Can you work these out from the drawing? Everything is in mm from the part's minimum corner. Coordinates: 2 decimals unless noted, no trailing zeros. Loops run counter-clockwise (first coordinate to the right, second up) from the corner with the lowest first, then second, coordinate; pieces in that order, holes last.
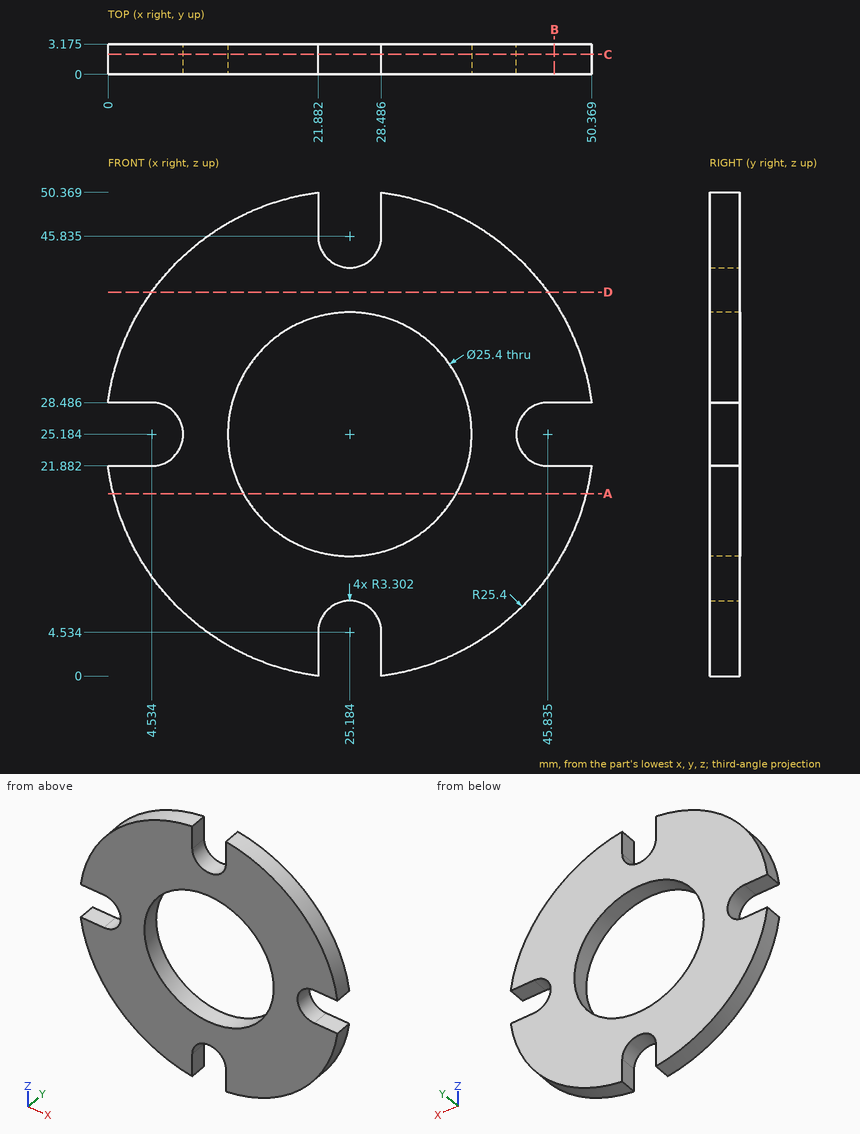
1. I want a section at D-D (z = 40). Please give me the cut outline in (x, y) (1 decimal).
2. I want a section at B-B (x = 46.5). Please give me the cut outline in (y, z) (1 decimal).
3. For pin 1 (1 mm diameter, centred on y = 2, z = 3, fed in from -X); pin 2 (1.6 mm diameter, centred on x = 47.5, y = 1, fed in from +Z) (1 decimal); pin 3 (1 mm diameter, centred on y = 2, z = 48, fed in from +X) (1 decimal); pin 4 (3 mm diameter, centred on x = 19, z = 35.5, fed in from +Y) (3 decimals), each with a flat end and sliding along its axis, tell me the tip position at first contact or that it passes through.
4. I need wall thicknesses on line 1 along Z through (x, y) = (25, 1.75) (1 decimal); line 2 along Z through (x, y) = (43, 0.45) (1 decimal); line 3 along X through (y, z) = (2.3, 17) (1 decimal). Which ranges of each line are inside material? Lowest first, please.
5. I want a section at C-C (y = 2.1). Please give me the cut outline in (x, z) (1 decimal), then the cut area to 3 significant figures.
6. I want a section at A-A (z = 19). Please give me the cut outline in (x, y) (1 decimal).
Response values:
1. outline: (4.6, 0) - (45.8, 0) - (45.8, 3.2) - (4.6, 3.2) - close
2. outline: (0, 11.4) - (3.2, 11.4) - (3.2, 21.9) - (0, 21.9) - close; (0, 28.5) - (3.2, 28.5) - (3.2, 39) - (0, 39) - close
3. pin 1: stops at x = 11.96
3. pin 2: stops at z = 38.7
3. pin 3: stops at x = 37.3
3. pin 4: stops at y = 3.175
4. line 1: z = 7.8 to 12.5, 37.9 to 42.5
4. line 2: z = 7.1 to 23.5, 26.9 to 43.3
4. line 3: x = 1.1 to 15.5, 34.9 to 49.2
5. outline: (0, 21.9) arc R25.4 ccw to (21.9, 0) - (21.9, 4.5) arc R3.3 cw to (28.5, 4.5) - (28.5, 0) arc R25.4 ccw to (50.4, 21.9) - (45.8, 21.9) arc R3.3 cw to (45.8, 28.5) - (50.4, 28.5) arc R25.4 ccw to (28.5, 50.4) - (28.5, 45.8) arc R3.3 cw to (21.9, 45.8) - (21.9, 50.4) arc R25.4 ccw to (0, 28.5) - (4.5, 28.5) arc R3.3 cw to (4.5, 21.9) - close; hole circle Ø25.4 at (25.2, 25.2)
5. area: 1,330 mm2
6. outline: (0.5, 0) - (14.1, 0) - (14.1, 3.2) - (0.5, 3.2) - close; (36.3, 0) - (49.8, 0) - (49.8, 3.2) - (36.3, 3.2) - close
